The figure shows three views and two pictorial views of one solid part (mm, origin at its lowest corner). Answer the questions. A direction names the side the tool comes from. Round coordinates to 2 decimals unless told otherwise and drop trailing zeros. Order: outer loops, then holes, each group sorted by start corner. A loop starts at its lowest first (then second) coordinate and runs counter-clockwise, first axis right, second up. Notation, with made-up numbers: M -24,83 L 9,83 A16 cw 9,92 Z; hole C -29,78.25 d10. An arc over 180 degrees is marked long. Return JSON: item names as keys, results as strings.
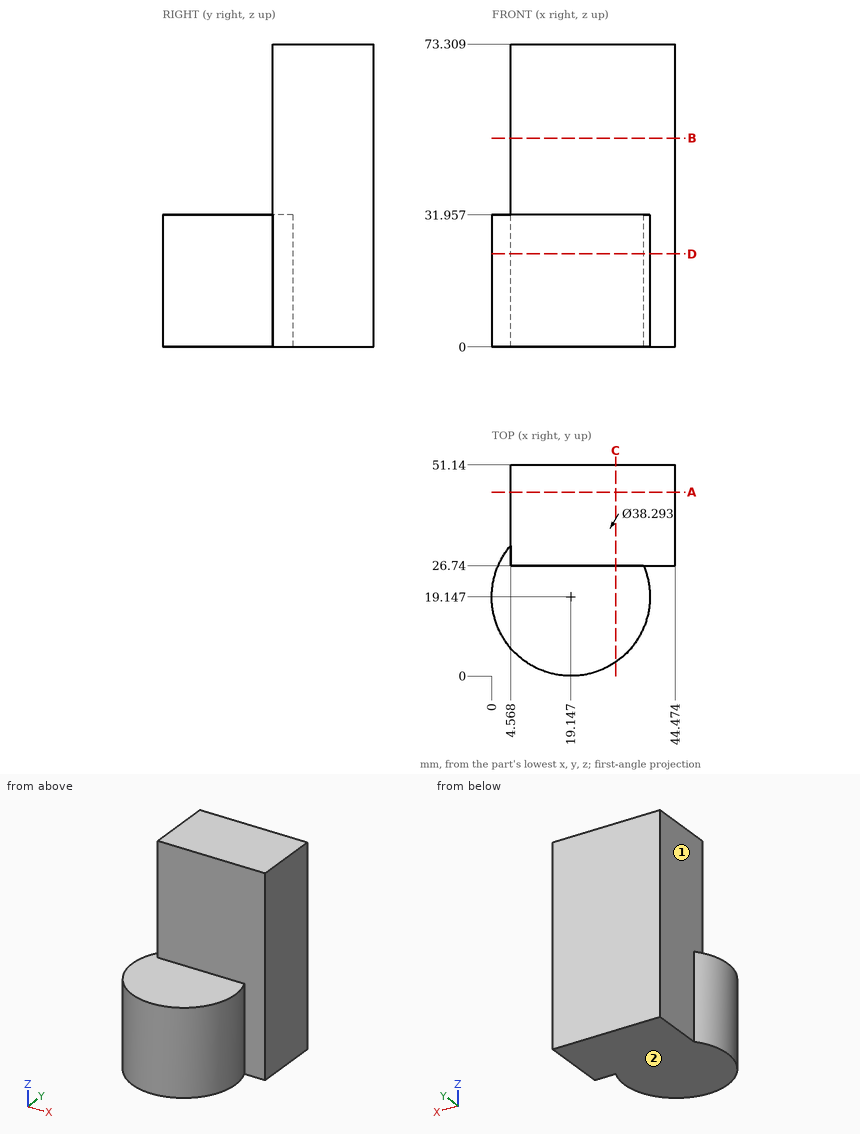
Item 1: Each of these flat-tipped pins is pushed along its axis until it touches: pin 1 (7.5 mm diameter, centred on y = 43.5, z = 27, fed in from -X); pin 2 (25 mm diameter, centred on x = 27, y = 8, fed in from +Z); pin 3 (4 mm diameter, centred on x = 30, z = 36, fed in from -Y). Where does it stop, or does it pass through?
Output:
{"pin 1": "stops at x = 4.57", "pin 2": "stops at z = 31.96", "pin 3": "stops at y = 26.74"}
Item 2: Find section D-D (z = 22.5). Determine the outline of the cut face in (x, y).
Output:
{"outline": "M 4.57,31.56 A19.15 ccw long 36.72,26.74 L 44.47,26.74 L 44.47,51.14 L 4.57,51.14 Z"}
Item 3: Consider line 1 along X through (y, z) = (44.5, 15); line 2 along Z through (x, y) = (3.5, 16); line 3 along Y through (x, z) = (43.5, 44). Determine where each line is inside the solid, lowest interval first. Write a range as [from, to].
Output:
{"line 1": "x = [4.57, 44.47]", "line 2": "z = [0, 31.96]", "line 3": "y = [26.74, 51.14]"}
Item 4: Find section B-B (z = 50.5). Determine the outline of the cut face in (x, y).
Output:
{"outline": "M 4.57,26.74 L 44.47,26.74 L 44.47,51.14 L 4.57,51.14 Z"}
Item 5: Find section A-A (y = 44.5). Determine the outline of the cut face in (x, z), plus the area to 3 significant figures.
Output:
{"outline": "M 4.57,0 L 44.47,0 L 44.47,73.31 L 4.57,73.31 Z", "area": "2,930 mm^2"}
Item 6: Which of the six approach directions +Z, -Z, +X, -X, +Y, -Y give full straight-line access (tool end or side, diameter ignored) to the marked faces 1 and 2?
Output:
{"face 1": "+Z, -X, +Y", "face 2": "-Z, +X, -X, +Y, -Y"}
Item 7: Find section C-C (x = 30). Determine the outline of the cut face in (y, z).
Output:
{"outline": "M 3.37,0 L 51.14,0 L 51.14,73.31 L 26.74,73.31 L 26.74,31.96 L 3.37,31.96 Z"}
